from build123d import *

# Parameters (mm, degrees)
F0_W     = 45
F0_H     = 83.05
F0_W_2   = 45.96
F1_DEPTH = 15
F2_DEPTH = 2.76
F3_W     = 45
F3_H     = 83.05
F4_DEPTH = 4
F5_R     = 7.300499
F6_DEPTH = 15.001


with BuildPart() as f1:
    # F0 (on Top) → F1 (new body)
    with BuildSketch(Plane.XY):
        with Locations((-45.48, 0)):
            Rectangle(F0_W, F0_H)
        with Locations((-0.48, 0)):
            Rectangle(F0_W, F0_H)
        with Locations((45, 0)):
            Rectangle(F0_W_2, F0_H)
    extrude(amount=-F1_DEPTH)

    # F0 (on Top) → F2 (join)
    with BuildSketch(Plane.XY):
        with Locations((-0.48, 0)):
            Rectangle(F0_W, F0_H)
    extrude(amount=F2_DEPTH)

    # F3 (on face) → F4 (cut)
    with BuildSketch(Plane(origin=(0, 0, -15), x_dir=(1, 0, 0), z_dir=(0, 0, -1))):
        with Locations((-0.48, 0)):
            Rectangle(F3_W, F3_H)
    extrude(amount=-F4_DEPTH, mode=Mode.SUBTRACT)

    # F5 (on face) → F6 (cut, through all)
    with BuildSketch(Plane.XY):
        with Locations((-47.45315, 29.645713)):
            Circle(F5_R)
        with Locations((-47.45315, -29.645713)):
            Circle(F5_R)
        with Locations((47.45315, 29.645713)):
            Circle(F5_R)
        with Locations((47.45315, -29.645713)):
            Circle(F5_R)
    extrude(amount=-F6_DEPTH, mode=Mode.SUBTRACT)


solid = f1.part
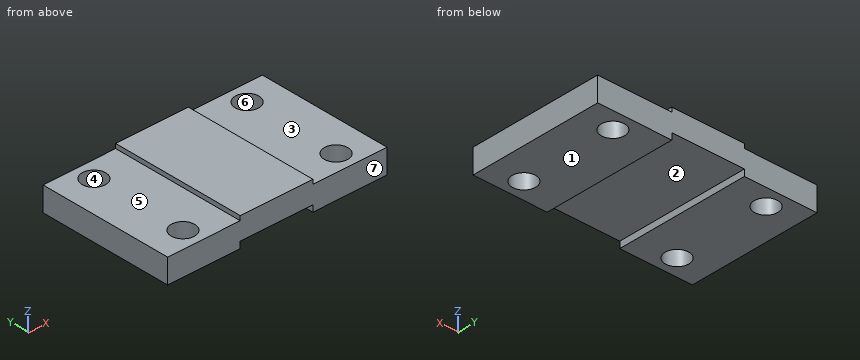
Source: CAD feature listing. Evaluate the final solid. Frame: model axes, mm. Face numbers are marked on the shaded views. A direction names the side the tool comes from. Round coordinates to 2 decimals unless told otherwise and drop trailing zeros. Loops run counter-clockwise (first coordinate to the right, second up) from the corner with the lowest first, then second, coordinate; pieces in that order, holes last. Notation, with made-up numbers: (21, 18.25) -> (80, 18.25) arc R17 cw to (80, 43.25) -> close; hole circle Ø6 at (-21, 11.25). An arc over 180 degrees is marked (long way). Answer as a JSON object with one key per item and string values. Group by question number.
Q1. Section query D-D (y = 31). Output: boundary loops of the cut face in (x, z), plus the area to 3 significant figures.
Q2. Mould query, pull axis Y, two halves, no side actions, for the marked faces 4, 5, 6 and 7. Classes: pulls with the +Y half, pulls with the -Y half, needs draft (parallel to the pull), parting line crosses it, or undercut.
Q3. Ray query, line 1 (X direction, y = -36, z = -3.5); line 2 (Z direction, x = -33, y = -3.5); line 3 (X direction, y = 19.5, z = -11.5). Return the intervals inside material, ascending. Write a range as from..to.
Q4. Section query C-C (x = -53). Output: boundary loops of the cut face in (y, z) (3 decimals).
Q5. Section query A-A (y = 14). Output: boundary loops of the cut face in (x, z).
Q6. Section query B-B (z = -12.5). Output: boundary loops of the cut face in (x, y) (1 decimal).
Q7. Contact query for flat-ended pins moving along their axis: P1, Ø3, axis at x = -40.5, y = 1.5, coming from the +Z side; P2, Ø1, axis at x = -7, y = 5, coming from the -Z side; P3, Ø1.4, axis at y = 7.5, z = 1, coming from the -X side. Output: stop coordinate, or through.
Q8. Access query for the marked faces 1, 2 and 3. Directions: +Z, -Z, +X, -X, +Y, -Y. A direction counts if a zero-diameter tool reaches every point of the face in a straight line with its end or side. Return the directions, or none.
Completed:
{
 "1": {"outline": "(-67.98, -15) -> (-54.63, -15) -> (-54.63, 0) -> (-67.98, 0) -> close; (-40.28, -15) -> (-22.98, -15) -> (-22.98, -11) -> (22.02, -11) -> (22.02, -15) -> (40.28, -15) -> (40.28, 0) -> (22.02, 0) -> (22.02, 2.76) -> (-22.98, 2.76) -> (-22.98, 0) -> (-40.28, 0) -> close; (54.63, -15) -> (67.98, -15) -> (67.98, 0) -> (54.63, 0) -> close", "area": "1,550 mm²"},
 "2": {"face 4": "undercut", "face 5": "needs draft", "face 6": "undercut", "face 7": "pulls with the -Y half"},
 "3": {"line 1": "-67.98..-51.05, -43.86..43.86, 51.05..67.98", "line 2": "-15..0", "line 3": "-67.98..-22.98, 22.02..67.98"},
 "4": {"outline": "(-41.525, -15) -> (-34.392, -15) -> (-34.392, 0) -> (-41.525, 0) -> close; (-24.899, -15) -> (24.899, -15) -> (24.899, 0) -> (-24.899, 0) -> close; (34.392, -15) -> (41.525, -15) -> (41.525, 0) -> (34.392, 0) -> close"},
 "5": {"outline": "(-67.98, -15) -> (-22.98, -15) -> (-22.98, -11) -> (22.02, -11) -> (22.02, -15) -> (67.98, -15) -> (67.98, 0) -> (22.02, 0) -> (22.02, 2.76) -> (-22.98, 2.76) -> (-22.98, 0) -> (-67.98, 0) -> close"},
 "6": {"outline": "(-68, -41.5) -> (-23, -41.5) -> (-23, 41.5) -> (-68, 41.5) -> close; (22, -41.5) -> (68, -41.5) -> (68, 41.5) -> (22, 41.5) -> close; hole circle Ø14.6 at (-47.5, -29.6); hole circle Ø14.6 at (-47.5, 29.6); hole circle Ø14.6 at (47.5, -29.6); hole circle Ø14.6 at (47.5, 29.6)"},
 "7": {"P1": "z = 0", "P2": "z = -11", "P3": "x = -22.98"},
 "8": {"face 1": "-Z, +X, -X, +Y, -Y", "face 2": "-Z, +Y, -Y", "face 3": "+Z, +X, +Y, -Y"}
}
